Design review of the part built by this model. Coordinates are the model's own, in mm. Face numbers are marked on the shaded views. Give positions to 0.01 mm unless a question says otherwise; leave off trailing zeros. Loops run counter-clockwise (first coordinate to the right, second up) from the corner with the lowest first, then second, coordinate; pieces in that order, holes last. Notation, with made-up numbers: (-31.5, -40) - (15.5, -40) arc R24 cw to (15.5, -27) - close; hole circle Ø11 at (63.5, 69.25). An arc over 180 degrees is marked (long way). One line per item, written item: value. Start each with the question number.
```python
from build123d import *

# Parameters (mm, degrees)
F2_R     = 9.000031
F3_DEPTH = 67.8
F5_R     = 2.197813
F6_DEPTH = 16.3


with BuildPart() as f1:
    # F0 (on Front) → F1 (revolve)
    with BuildSketch(Plane.XZ):
        Polygon((0, 3.423913), (0, 0), (42.65625, 0), (46.650816, 0), (46.650816, 34.018698), (60.346473, 28.247284), (46.650816, 36.807068), (0, 60.774457), (0, 54.78261), (42.65625, 36.807068), (42.65625, 3.423913), align=None)
    revolve(axis=Axis((0, 0, 1.711957), (0, 0, 1)))

    # F2 (on Front) → F3 (cut)
    with BuildSketch(Plane.XZ):
        with Locations((0, 15.407609)):
            Circle(F2_R)
    extrude(amount=F3_DEPTH, mode=Mode.SUBTRACT)

    # F5 (on offset) → F6 (join)
    with BuildSketch(Plane.XZ.offset(45.8)):
        with Locations((0, 4.250792)):
            Circle(F5_R)
    extrude(amount=F6_DEPTH)


solid = f1.part
```
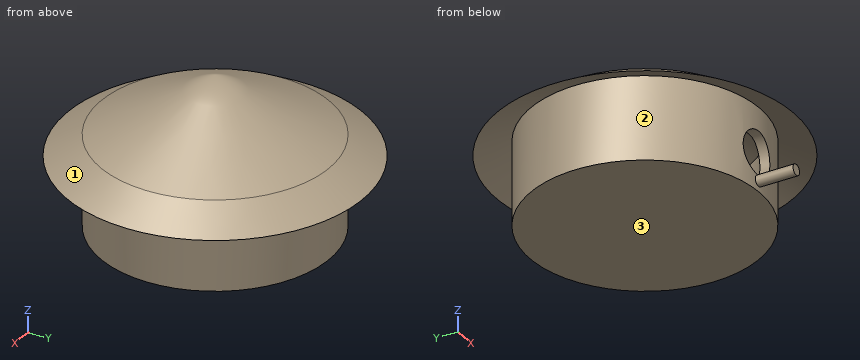
(1) For pin 1 Ø4 at (y, z) = (43, 28.5) entering from +X; pin 2 Ø5 at (x, y) = (-45.5, 8) entering from +Z; pin 3 Ø10 at (x, z) = (-23.5, 12) entering from -Y, all flat-tipped, find the tip position at first contact; note any pin that passes through.
(2) Take a section at C-C on z = 41. State the section outline as (x, y) points, and give its area (3 significant figures).
(3) Take a section at B-B on z = 57. State the section outline as (x, y) points, and give its area (3 significant figures).
(4) Take a section at A-A on z = 26.5. State the section outline as (x, y) points.
(5) Draft analysis for pull direction Y (two halves, no side actions). For the marked faces 1, 2 and 3, state which applies: pulls with the +Y half, pulls with the -Y half, needs draft (parallel to the pull), parting line crosses it, or undercut.
(6) To check wall thickness, follow L1, parallel to Y at x = 0, z = 27; L2, parallel to Z at x = 0, y = -43.85; L3, parallel to Z at x = -19.5, y = 11. State the ranges of each line that lie inside material, in increasing order. Write a range as from..to.
(7) Take a section at D-D on z = 12. State the section outline as (x, y) points (1 decimal).
Here are the results:
1. pin 1: x = 44.26
1. pin 2: z = 38.32
1. pin 3: y = -42.83
2. outline: circle Ø76.98 at (0, 0); hole circle Ø65.41 at (0, 0)
2. area: 1,290 mm²
3. outline: circle Ø14.69 at (0, 0)
3. area: 170 mm²
4. outline: circle Ø93.3 at (0, 0); hole circle Ø85.31 at (0, 0)
5. face 1: parting line crosses it
5. face 2: undercut
5. face 3: needs draft
6. L1: -46.65..-42.66, 42.66..46.65
6. L2: 0..6.41, 24.41..38.25
6. L3: 0..3.42, 45.35..49.27
7. outline: (-8.3, -45.9) - (-8.3, -41.8) arc R42.7 cw (long way) to (8.3, -41.8) - (8.3, -45.9) arc R46.7 ccw (long way) to start
